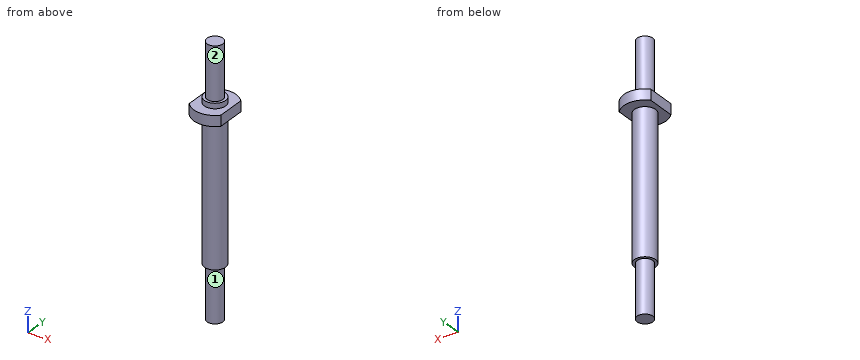
```python
from build123d import *

# Parameters (mm, degrees)
EXTRUDE_1_DEPTH = 2
SKETCH_2_R      = 2
EXTRUDE_2_DEPTH = 1
SKETCH_3_R      = 1.5
EXTRUDE_3_DEPTH = 10
EXTRUDE_START   = 27
SKETCH_4_R      = 2
EXTRUDE_4_DEPTH = 27
EXTRUDE_START_2 = 10
SKETCH_5_R      = 1.5
EXTRUDE_5_DEPTH = 10


with BuildPart() as part:
    # 草图1 → 凸台-拉伸1 (new body)
    with BuildSketch(Plane.XY):
        with BuildLine():
            Line((-3, 2.645751311), (-3, -2.645751311))
            ThreePointArc((-3, -2.645751311), (0, -4), (3, -2.645751311))
            Line((3, -2.645751311), (3, 2.645751311))
            ThreePointArc((3, 2.645751311), (0, 4), (-3, 2.645751311))
        make_face()
    extrude(amount=EXTRUDE_1_DEPTH)

    # 草图2 → 凸台-拉伸2 (add)
    with BuildSketch(Plane.XY.offset(2)):
        Circle(SKETCH_2_R)
    extrude(amount=EXTRUDE_2_DEPTH)

    # 草图3 → 凸台-拉伸3 (add)
    with BuildSketch(Plane.XY.offset(3)):
        Circle(SKETCH_3_R)
    extrude(amount=EXTRUDE_3_DEPTH)

    # 草图4 → 凸台-拉伸4 (add)
    with BuildSketch(Plane(origin=(0, 0, 0), x_dir=(-1, 0, 0), z_dir=(0, 0, -1)).offset(EXTRUDE_START)):
        with Locations(Location((0, 0, 0), (0, 0, 180))):
            Circle(SKETCH_4_R)
    extrude(amount=-EXTRUDE_4_DEPTH)

    # 草图5 → 凸台-拉伸5 (add)
    with BuildSketch(Plane(origin=(0, 0, -27), x_dir=(-1, 0, 0), z_dir=(0, 0, -1)).offset(EXTRUDE_START_2)):
        with Locations(Location((0, 0, 0), (0, 0, 180))):
            Circle(SKETCH_5_R)
    extrude(amount=-EXTRUDE_5_DEPTH)


solid = part.part
```
The listing builds one solid part. Answer for the finished solid, in the listing's coordinates (mm). Face numbers are marked on the shaded views. A direction names the side the tool comes from. Round coordinates to 2 decimals unless told otherwise and drop trailing zeros. Loops run counter-clockwise (first coordinate to the right, second up) from the corner with the lowest first, then second, coordinate; pieces in that order, holes last.
Q1. Section D-D, the plane z = 8 is taken. Determine the outline of the cut face in (x, y), then the cut area to 3 significant figures.
Q2. Which of the six approach directions +Z, -Z, +X, -X, +Y, -Y give full straight-line access (tool end or side, diameter ignored) to the marked faces 1 and 2?
Q3. Section B-B, the plane y = 0 is taken. Determine the outline of the cut face in (x, z), then the cut area to 3 significant figures.
Q4. Section C-C, the plane z = -24 is taken. Determine the outline of the cut face in (x, y), then the cut area to 3 significant figures.
Q5. Given pin 1 Ø1 at (x, z) = (2, -22.5) entering from -Y; pin 2 Ø1.5 at (x, z) = (0, -6.5) entering from +Y; pin 3 Ø2 at (x, y) = (-1, -2.5) entering from +Z, each flat-ended and moving along its own axis, determine where each tip first touches the part or whether it passes through.
Q6. Find the intervals of material crossed by line 1 (Z direction, x = 0.5, y = -2.5); line 2 (Y direction, x = 0, z = -27.5); line 3 (Z direction, x = -1.5, y = 1), in increasing order.
Q7. Section A-A, the plane x = 0 is taken. Determine the outline of the cut face in (y, z), then the cut area to 3 significant figures.
Completed:
1. outline: circle Ø3 at (0, 0)
1. area: 7.07 mm2
2. face 1: -Z
2. face 2: +Z
3. outline: (-3, 0) - (-2, 0) - (-2, -27) - (-1.5, -27) - (-1.5, -37) - (1.5, -37) - (1.5, -27) - (2, -27) - (2, 0) - (3, 0) - (3, 2) - (2, 2) - (2, 3) - (1.5, 3) - (1.5, 13) - (-1.5, 13) - (-1.5, 3) - (-2, 3) - (-2, 2) - (-3, 2) - close
3. area: 184 mm2
4. outline: circle Ø4 at (0, 0)
4. area: 12.6 mm2
5. pin 1: stops at y = -1.32
5. pin 2: stops at y = 2
5. pin 3: stops at z = 3
6. line 1: z = 0 to 2
6. line 2: y = -1.5 to 1.5
6. line 3: z = -27 to 3
7. outline: (-4, 0) - (-2, 0) - (-2, -27) - (-1.5, -27) - (-1.5, -37) - (1.5, -37) - (1.5, -27) - (2, -27) - (2, 0) - (4, 0) - (4, 2) - (2, 2) - (2, 3) - (1.5, 3) - (1.5, 13) - (-1.5, 13) - (-1.5, 3) - (-2, 3) - (-2, 2) - (-4, 2) - close
7. area: 188 mm2
